Source: CAD feature listing. Evaluate the final solid. Frame: model axes, mm. Face numbers are marked on the shaded views. A direction names the side the tool comes from. Coordinates: 2 decimals unless noted, no trailing zeros. Write each loop counter-clockwise with the first axis right and the second up, starting at its lowest first coordinate (ties: lowest second). Pieces come first, ordered by that corner, then holes. Notation, with made-up numbers: (4.25, 3) -> (25.25, 3) arc R24 ccw to (25.25, 24) -> close; hole circle Ø3 at (70.5, 59.25). An arc over 180 degrees is marked (long way). Write item = value, one per line.
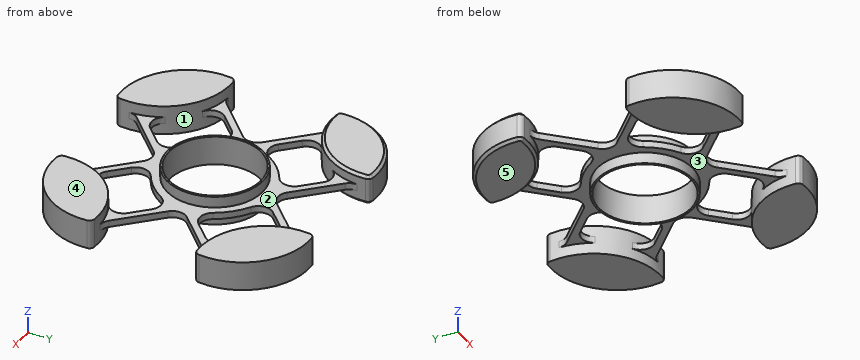
from build123d import *

# Parameters (mm, degrees)
F0_R     = 11.43
F1_DEPTH = 0.79375
F2_R     = 11.43
F2_R_2   = 10.9855
F3_DEPTH = 3.4798
F5_DEPTH = 3.4798
F6_R     = 3.175
F7_SIZE  = 0.635


# Not quite as in the source:
# - a feature names something its author has since deleted; it is built from what else it names


with BuildPart() as f1:
    # F0 (on Top) → F1 (new body, symmetric)
    with BuildSketch(Plane.XY):
        Polygon((-14.3684097937, 28.0844097937), (-28.2927262655, 14.5767262655), (-13.716, 0), (-28.0844097937, -14.3684097937), (-14.5767262655, -28.2927262655), (0, -13.716), (14.3684097937, -28.0844097937), (28.2927262655, -14.5767262655), (13.716, 0), (28.0844097937, 14.3684097937), (14.5767262655, 28.2927262655), (0, 13.716), align=None)
        with BuildLine():
            ThreePointArc((-13.0320412256, -24.4131746341), (-20.1396997698, -20.0947125947), (-24.2403197525, -12.8591863439))
            Line((-24.2403197525, -12.8591863439), (-13.5538149684, -2.1726815599))
            ThreePointArc((-13.5538149684, -2.1726815599), (-9.4531949857, -9.4082078106), (-2.3455364415, -13.72666985))
            Line((-2.3455364415, -13.72666985), (-13.0320412256, -24.4131746341))
        make_face(mode=Mode.SUBTRACT)
        with BuildLine():
            ThreePointArc((24.4131746341, -13.0320412256), (20.0947125947, -20.1396997698), (12.8591863439, -24.2403197525))
            Line((12.8591863439, -24.2403197525), (2.1726815599, -13.5538149684))
            ThreePointArc((2.1726815599, -13.5538149684), (9.4082078106, -9.4531949857), (13.72666985, -2.3455364415))
            Line((13.72666985, -2.3455364415), (24.4131746341, -13.0320412256))
        make_face(mode=Mode.SUBTRACT)
        Circle(F0_R, mode=Mode.SUBTRACT)
        with BuildLine():
            ThreePointArc((-2.1726815599, 13.5538149684), (-9.4082078106, 9.4531949857), (-13.72666985, 2.3455364415))
            Line((-13.72666985, 2.3455364415), (-24.4131746341, 13.0320412256))
            ThreePointArc((-24.4131746341, 13.0320412256), (-20.0947125947, 20.1396997698), (-12.8591863439, 24.2403197525))
            Line((-12.8591863439, 24.2403197525), (-2.1726815599, 13.5538149684))
        make_face(mode=Mode.SUBTRACT)
        with BuildLine():
            ThreePointArc((13.0320412256, 24.4131746341), (20.1396997698, 20.0947125947), (24.2403197525, 12.8591863439))
            Line((24.2403197525, 12.8591863439), (13.5538149684, 2.1726815599))
            ThreePointArc((13.5538149684, 2.1726815599), (9.4531949857, 9.4082078106), (2.3455364415, 13.72666985))
            Line((2.3455364415, 13.72666985), (13.0320412256, 24.4131746341))
        make_face(mode=Mode.SUBTRACT)
    extrude(amount=F1_DEPTH, both=True)

    # F2 (on Top) → F3 (join, symmetric)
    with BuildSketch(Plane.XY):
        Circle(F2_R)
        Circle(F2_R_2, mode=Mode.SUBTRACT)
    extrude(amount=F3_DEPTH, both=True)

    # F4 (on Top) → F5 (join, symmetric)
    with BuildSketch(Plane.XY):
        with BuildLine():
            ThreePointArc((-13.1605476158, 30.3918186243), (-25.856934394, 25.9965462925), (-30.6357520227, 13.4394941638))
            ThreePointArc((-30.6357520227, 13.4394941638), (-30.5278746276, 13.0126091951), (-30.2807216131, 12.6482142222))
            Line((-30.2807216131, 12.6482142222), (-12.3804144461, 30.0129218371))
            ThreePointArc((-12.3804144461, 30.0129218371), (-12.7371356357, 30.2710270515), (-13.1605476158, 30.3918186243))
        make_face()
        with BuildLine():
            Line((-12.3804144461, 30.0129218371), (-30.2807216131, 12.6482142222))
            ThreePointArc((-30.2807216131, 12.6482142222), (-29.9240004235, 12.3901090077), (-29.5005884435, 12.2693174349))
            ThreePointArc((-29.5005884435, 12.2693174349), (-16.8042016652, 16.6645897667), (-12.0253840365, 29.2216418954))
            ThreePointArc((-12.0253840365, 29.2216418954), (-12.1332614316, 29.6485268641), (-12.3804144461, 30.0129218371))
        make_face()
        with BuildLine():
            ThreePointArc((-30.3918186243, -13.1605476158), (-25.9965462925, -25.856934394), (-13.4394941638, -30.6357520227))
            ThreePointArc((-13.4394941638, -30.6357520227), (-13.0126091951, -30.5278746276), (-12.6482142222, -30.2807216131))
            Line((-12.6482142222, -30.2807216131), (-30.0129218371, -12.3804144461))
            ThreePointArc((-30.0129218371, -12.3804144461), (-30.2710270515, -12.7371356357), (-30.3918186243, -13.1605476158))
        make_face()
        with BuildLine():
            Line((-30.0129218371, -12.3804144461), (-12.6482142222, -30.2807216131))
            ThreePointArc((-12.6482142222, -30.2807216131), (-12.3901090077, -29.9240004235), (-12.2693174349, -29.5005884435))
            ThreePointArc((-12.2693174349, -29.5005884435), (-16.6645897667, -16.8042016652), (-29.2216418954, -12.0253840365))
            ThreePointArc((-29.2216418954, -12.0253840365), (-29.6485268641, -12.1332614316), (-30.0129218371, -12.3804144461))
        make_face()
        with BuildLine():
            ThreePointArc((13.1605476158, -30.3918186243), (25.856934394, -25.9965462925), (30.6357520227, -13.4394941638))
            ThreePointArc((30.6357520227, -13.4394941638), (30.5278746276, -13.0126091951), (30.2807216131, -12.6482142222))
            Line((30.2807216131, -12.6482142222), (12.3804144461, -30.0129218371))
            ThreePointArc((12.3804144461, -30.0129218371), (12.7371356357, -30.2710270515), (13.1605476158, -30.3918186243))
        make_face()
        with BuildLine():
            Line((12.3804144461, -30.0129218371), (30.2807216131, -12.6482142222))
            ThreePointArc((30.2807216131, -12.6482142222), (29.9240004235, -12.3901090077), (29.5005884435, -12.2693174349))
            ThreePointArc((29.5005884435, -12.2693174349), (16.8042016652, -16.6645897667), (12.0253840365, -29.2216418954))
            ThreePointArc((12.0253840365, -29.2216418954), (12.1332614316, -29.6485268641), (12.3804144461, -30.0129218371))
        make_face()
        with BuildLine():
            ThreePointArc((30.3918186243, 13.1605476158), (25.9965462925, 25.856934394), (13.4394941638, 30.6357520227))
            ThreePointArc((13.4394941638, 30.6357520227), (13.0126091951, 30.5278746276), (12.6482142222, 30.2807216131))
            Line((12.6482142222, 30.2807216131), (30.0129218371, 12.3804144461))
            ThreePointArc((30.0129218371, 12.3804144461), (30.2710270515, 12.7371356357), (30.3918186243, 13.1605476158))
        make_face()
        with BuildLine():
            Line((30.0129218371, 12.3804144461), (12.6482142222, 30.2807216131))
            ThreePointArc((12.6482142222, 30.2807216131), (12.3901090077, 29.9240004235), (12.2693174349, 29.5005884435))
            ThreePointArc((12.2693174349, 29.5005884435), (16.6645897667, 16.8042016652), (29.2216418954, 12.0253840365))
            ThreePointArc((29.2216418954, 12.0253840365), (29.6485268641, 12.1332614316), (30.0129218371, 12.3804144461))
        make_face()
    extrude(amount=F5_DEPTH, both=True)

    # F6
    f6_edges = [f1.edges().sort_by_distance(p)[0] for p in [
        (-26.008197, 12.292197, 0),
        (-12.533339, 23.914473, 0),
        (-24.032883, 12.65175, 0),
        (-12.136817, 25.852817, 0),
        (-2.172682, 13.553815, 0),
        (-13.72667, 2.345536, 0),
        (-13.716, 0, 0),
        (0, 13.716, 0),
        (2.345536, 13.72667, 0),
        (13.553815, 2.172682, 0),
        (13.716, 0, 0),
        (13.72667, -2.345536, 0),
        (2.172682, -13.553815, 0),
        (0, -13.716, 0),
        (-2.345536, -13.72667, 0),
        (-13.553815, -2.172682, 0),
        (12.292197, 26.008197, 0),
        (12.65175, 24.032883, 0),
        (25.852817, 12.136817, 0),
        (23.914473, 12.533339, 0),
        (26.008197, -12.292197, 0),
        (24.032883, -12.65175, 0),
        (12.136817, -25.852817, 0),
        (12.533339, -23.914473, 0),
        (-12.292197, -26.008197, 0),
        (-12.65175, -24.032883, 0),
        (-25.852817, -12.136817, 0),
        (-23.914473, -12.533339, 0),
    ]]
    fillet(f6_edges, radius=F6_R)

    # F7
    f7_edges = [f1.edges().sort_by_distance(p)[0] for p in [
        (-25.856934, 25.996546, 3.4798),
        (-30.280722, 12.648214, 3.4798),
        (-16.804202, 16.66459, 3.4798),
        (-12.380414, 30.012922, 3.4798),
        (-25.856934, 25.996546, -3.4798),
        (-30.280722, 12.648214, -3.4798),
        (-16.804202, 16.66459, -3.4798),
        (-12.380414, 30.012922, -3.4798),
    ]]
    chamfer(f7_edges, length=F7_SIZE)


solid = f1.part
1) First-contact query: pin 1 Ø16.5 at (x, y) = (8.5, -5.5) entering from -Z; pin 2 Ø2 at (y, z) = (19, 0.5) entering from +X; pin 3 Ø6 at (x, y) = (17.5, 1.5) entering from -Z; pin 4 Ø4 at (y, z) = (-1.5, 1.5) entering from +X. Flat tips, straight axial feed; report the tip coordinate or a pass-through.
Answer block:
pin_1 = -3.48
pin_2 = 30.15
pin_3 = -0.79
pin_4 = 17.09
2) Reachability of the marked faces 1, 2, 3, 4 and 5 from +Z, -Z, +X, -X, +Y, -Y: full face, straight path, thin tool, end or side. Return the list, or none.
Answer block:
face_1 = none
face_2 = +Z
face_3 = -Z
face_4 = +Z, +X, -X, +Y, -Y
face_5 = -Z, +X, -X, +Y, -Y
3) Material intervals for probe 1 along Y at (x, z) = (0, 0.5); probe 2 along Y at (x, z) = (-19, 0.25); probe 3 along Y at (x, z) = (-13.5, 3), sorted ascending. Write a range as [from, to].
Answer block:
probe_1 = [-15.03, -10.99], [10.99, 15.03]
probe_2 = [-30.06, -14.82], [-7.62, -5.28], [5.28, 7.62], [14.89, 29.91]
probe_3 = [-30.64, -21.53], [21.66, 30.27]
4) Cut plane D-D, the plane x = -10. Output: boundary loops of the cut face in (y, z).
Answer block:
outline = (-23.72, -0.79) -> (-21.2, -0.79) -> (-21.2, 0.79) -> (-23.72, 0.79) -> close; (-8.82, -0.79) -> (-5.54, -0.79) -> (-5.54, -3.48) -> (-4.55, -3.48) -> (-4.55, 3.48) -> (-5.54, 3.48) -> (-5.54, 0.79) -> (-8.82, 0.79) -> close; (4.55, -3.48) -> (5.54, -3.48) -> (5.54, -0.79) -> (8.85, -0.79) -> (8.85, 0.79) -> (5.54, 0.79) -> (5.54, 3.48) -> (4.55, 3.48) -> close; (21.17, -0.79) -> (23.72, -0.79) -> (23.72, 0.79) -> (21.17, 0.79) -> close
5) Cut plane B-B, the plane x = 0. Output: boundary loops of the cut face in (y, z).
Answer block:
outline = (-15.03, -0.79) -> (-11.43, -0.79) -> (-11.43, -3.48) -> (-10.99, -3.48) -> (-10.99, 3.48) -> (-11.43, 3.48) -> (-11.43, 0.79) -> (-15.03, 0.79) -> close; (10.99, -3.48) -> (11.43, -3.48) -> (11.43, -0.79) -> (15.03, -0.79) -> (15.03, 0.79) -> (11.43, 0.79) -> (11.43, 3.48) -> (10.99, 3.48) -> close
6) Cut plane A-A, the plane z = 1.75. Give the number of separate pieces and of enclosed holes in the cut face, and give its area (3 significant figures).
Answer block:
separate_pieces = 5
enclosed_holes = 1
area = 962 mm2
